from build123d import *

# Parameters (mm, degrees)
CROQUIS1_W              = 250
CROQUIS1_H              = 250
SALIENTE_EXTRUIR1_DEPTH = 6
SALIENTE_EXTRUIR2_DEPTH = 30
REDONDEO1_R             = 3
CORTAR_EXTRUIR1_REACH   = 279.391
CROQUIS3_W              = 12
CROQUIS3_H              = 17
CROQUIS4_R              = 1
SALIENTE_EXTRUIR3_DEPTH = 3


with BuildPart() as part:
    # Croquis1 → Saliente-Extruir1 (new body)
    with BuildSketch(Plane(origin=(0, 0, 0), x_dir=(1, 0, 0), z_dir=(0, 1, 0))):
        Rectangle(CROQUIS1_W, CROQUIS1_H)
    extrude(amount=SALIENTE_EXTRUIR1_DEPTH)

    # Croquis2 → Saliente-Extruir2 (add)
    with BuildSketch(Plane(origin=(0, 6, 0), x_dir=(1, 0, 0), z_dir=(0, 1, 0))):
        Polygon((-120, 120), (-120, 90), (-117.5, 90), (-117.5, 117.5), (-90, 117.5), (-90, 120), align=None)
        Polygon((120, 120), (90, 120), (90, 117.5), (117.5, 117.5), (117.5, 90), (120, 90), align=None)
        Polygon((120, -120), (120, -90), (117.5, -90), (117.5, -117.5), (90, -117.5), (90, -120), align=None)
        Polygon((-120, -120), (-120, -90), (-117.5, -90), (-117.5, -117.5), (-90, -117.5), (-90, -120), align=None)
    extrude(amount=SALIENTE_EXTRUIR2_DEPTH)

    # Redondeo1
    redondeo1_edges = [part.edges().sort_by_distance(p)[0] for p in [
        (-118.75, 6, -90),
        (-117.5, 6, -103.75),
        (-103.75, 6, -117.5),
        (-90, 6, -118.75),
        (90, 6, -118.75),
        (103.75, 6, -117.5),
        (117.5, 6, -103.75),
        (118.75, 6, -90),
        (118.75, 6, 90),
        (117.5, 6, 103.75),
        (103.75, 6, 117.5),
        (90, 6, 118.75),
        (-90, 6, 118.75),
        (-103.75, 6, 117.5),
        (-117.5, 6, 103.75),
        (-118.75, 6, 90),
    ]]
    fillet(redondeo1_edges, radius=REDONDEO1_R)

    # Croquis3 → Cortar-Extruir1 (cut, up to next)
    with BuildSketch(Plane.XY.offset(120), mode=Mode.PRIVATE) as cortar_extruir1_sk1:
        Polygon((-102, 36), (-102, 19), (-90, 19.15390734), (-90, 36), align=None)
    cortar_extruir1_tool1 = extrude(cortar_extruir1_sk1.sketch, amount=-CORTAR_EXTRUIR1_REACH, mode=Mode.PRIVATE) & part.part
    # Croquis3 → Cortar-Extruir1 (cut, up to next)
    with BuildSketch(Plane.XY.offset(120), mode=Mode.PRIVATE) as cortar_extruir1_sk2:
        with Locations((96, 27.5)):
            Rectangle(CROQUIS3_W, CROQUIS3_H)
    cortar_extruir1_tool2 = extrude(cortar_extruir1_sk2.sketch, amount=-CORTAR_EXTRUIR1_REACH, mode=Mode.PRIVATE) & part.part
    add(cortar_extruir1_tool1.solids().sort_by_distance((-96.009095, 27.538419, 120))[0], mode=Mode.SUBTRACT)
    add(cortar_extruir1_tool2.solids().sort_by_distance((96, 27.5, 120))[0], mode=Mode.SUBTRACT)

    # Croquis4 → Saliente-Extruir3 (add)
    with BuildSketch(Plane(origin=(0, 6, 0), x_dir=(1, 0, 0), z_dir=(0, 1, 0))):
        with Locations(Location((0, 0, 0), (0, 0, 270))):
            Circle(CROQUIS4_R)
    extrude(amount=SALIENTE_EXTRUIR3_DEPTH)


solid = part.part
Input: part model. Units: mm. Frame: model coordinates. A direction names the side the tool comes from. Coordinates: 2 decimals unless noted, no trailing zeros. Order: outer loops, then holes, each group sorted by start corner. A loop starts at its lowest first (then second) coordinate and runs counter-clockwise, first axis right, second up. Notation, with made-up numbers: M -0.5,43.5 L 32.5,43.5 A18 cw 32.5,68.5 Z; hole C 2.25,-8 d4. An arc over 180 degrees is marked long. Answer as CSV lines item,"result".
1. Material intervals for line 1 (Z direction, x = 102.5, y = 25); line 2 (Y direction, x = -101, z = 32.5), sorted ascending. Write a range as from..to.
Reported:
line 1,"-120..-117.5, 117.5..120"
line 2,"0..6"
2. Section D-D (x = -11). Return the cut outline in (y, z), then the cut area to 3 significant figures.
Reported:
outline,"M 0,-125 L 6,-125 L 6,125 L 0,125 Z"
area,"1,500 mm2"
3. Access query for faces 4 (the flat face through (107, 19, 117.5)), 5 (the flat face through (-107, 17, 120)), 6 (the flat face through (-103, 21, -120)). Directions: +Z, -Z, +X, -X, +Y, -Y. A direction counts if a zero-diameter tool reaches every point of the face in a straight line with its end or side. Return the directions, or none.
Reported:
face 4,"+Y"
face 5,"+Z, +X, -X, +Y"
face 6,"-Z, +X, -X, +Y"
4. First-contact query: P1, Ø9, axis at x = -106.5, y = 22, coming from the -Z side; P2, Ø9, axis at x = -97.5, y = 18.5, coming from the +Z side; P3, Ø15, axis at y = 19.5, z = -102, coming from the +X side. Flat tips, straight axial feed; report the tip coordinate or a pass-through.
Reported:
P1,"z = -120"
P2,"z = 120"
P3,"x = 120"
5. Section B-B (x = 94.5). Return the cut outline in (y, z).
Reported:
outline,"M 0,-125 L 6,-125 L 6,-120 L 36,-120 L 36,-117.5 L 9,-117.5 A3 cw 6,-114.5 L 6,114.5 A3 cw 9,117.5 L 19,117.5 L 19,120 L 6,120 L 6,125 L 0,125 Z"
6. Pull-direction query (X, two-part tool) for faces 1 (the flat face through (120, 21, -103)), 2 (the flat face through (-2, 6, -2)), 3 (the flat face through (-118, 36, 109)); classes: released by +X, released by -X, zero draft, split by the parting line, or undercut.
Reported:
face 1,"released by +X"
face 2,"undercut"
face 3,"zero draft"
7. Section C-C (z = -63.5). Return the cut outline in (x, y).
Reported:
outline,"M -125,0 L 125,0 L 125,6 L -125,6 Z"
8. Section A-A (y = 31). Return the cut outline in (x, z).
Reported:
outline,"M -120,-120 L -90,-120 L -90,-117.5 L -117.5,-117.5 L -117.5,-90 L -120,-90 Z; M -120,90 L -117.5,90 L -117.5,117.5 L -102,117.5 L -102,120 L -120,120 Z; M 90,-120 L 120,-120 L 120,-90 L 117.5,-90 L 117.5,-117.5 L 90,-117.5 Z; M 102,117.5 L 117.5,117.5 L 117.5,90 L 120,90 L 120,120 L 102,120 Z"
